Check sheet for the modelled part. Datum: model origin and axes. Units: mm. A direction names the side the tool comes from. Give positions to 0.01 mm unless a question says otherwise; leave off trailing zeros. Write each loop counter-clockwise with the first axis right and the second up, starting at its lowest first coordinate (ties: lowest second). Pieces come first, ordered by that corner, then holes. Notation, with made-up numbers: M 2,31 L 21,31 A38 ccw 21,70 Z; hole C 49,0.5 d4. An arc over 180 degrees is marked long. Use CSV: the item, a comma, the result in double quotes. Start each with the question number.
1. Cross-section at B-B, the plane z = -12.5. Enter the section's corners in (x, y).
2. Access from +Z, -Z, +X, -X, +Y, -Y to the whole of each face (thin tool, end or side, straight path). Record for faces 1 (the face through (0, 0, -1)), 2 (the face through (1, 2, 32.625)).
3. Cross-section at C-C, the plane y = 1.5. State how many separate pieces and enclosed holes the cut face has, and give its area (3 significant figures).
4. Scan lines: line 1 (X direction, y = 2, z = 35); line 2 (Z direction, x = 32, y = 2.05); line 3 (X direction, y = 1, z = 13.5). Record each from-to range of solid material in increasing order.
5. Mould release check, pull along Z, two halves, no side actions. Record for faces 3 (the face through (1, 1, -54.875)), 4 (the face through (51.36, 1.48, 50.85)), 5 (the face through (10.14, 1.52, -14.8)): +Z half, -Z half, draft (parallel to the pull), parting line (faces both ways), or undercut.
6. Cross-section at A-A, the plane z = -28.5. Enter the section's corners in (x, y), and give its area (3 significant figures).
from build123d import *

# Parameters (mm, degrees)
SKETCH1_R           = 3
BOSS_EXTRUDE1_DEPTH = 3
SKETCH2_W           = 28
SKETCH2_H           = 5
SKETCH2_W_2         = 35.5
CUT_EXTRUDE1_DEPTH  = 79.545892535
CUT_EXTRUDE2_DEPTH  = 79.545892535
FILLET1_R           = 1.5
SKETCH4_W           = 28
SKETCH4_H           = 5
CUT_EXTRUDE3_DEPTH  = 79.545892535


with BuildPart() as part:
    # Sketch1 → Boss-Extrude1 (new body)
    with BuildSketch(Plane(origin=(0, 0, 0), x_dir=(1, 0, 0), z_dir=(0, 1, 0))):
        with BuildLine():
            Line((55.872458647, -40.12463695), (55.872458647, 39.87536305))
            ThreePointArc((55.872458647, 39.87536305), (51.479060365, 50.481964768), (40.872458647, 54.87536305))
            Line((40.872458647, 54.87536305), (-39.127541353, 54.87536305))
            ThreePointArc((-39.127541353, 54.87536305), (-49.734143071, 50.481964768), (-54.127541353, 39.87536305))
            Line((-54.127541353, 39.87536305), (-54.127541353, -40.12463695))
            ThreePointArc((-54.127541353, -40.12463695), (-49.734143071, -50.731238667), (-39.127541353, -55.12463695))
            Line((-39.127541353, -55.12463695), (40.872458647, -55.12463695))
            ThreePointArc((40.872458647, -55.12463695), (51.479060365, -50.731238667), (55.872458647, -40.12463695))
        make_face()
        with Locations(Location((48.872458647, 32.87536305, 0), (0, 0, 270))):
            Circle(SKETCH1_R, mode=Mode.SUBTRACT)
        with Locations(Location((-47.127541353, -33.12463695, 0), (0, 0, 270))):
            Circle(SKETCH1_R, mode=Mode.SUBTRACT)
        with Locations(Location((-32.127541353, -48.12463695, 0), (0, 0, 270))):
            Circle(SKETCH1_R, mode=Mode.SUBTRACT)
        with Locations(Location((33.872458647, -48.12463695, 0), (0, 0, 270))):
            Circle(SKETCH1_R, mode=Mode.SUBTRACT)
        with Locations(Location((48.872458647, -33.12463695, 0), (0, 0, 270))):
            Circle(SKETCH1_R, mode=Mode.SUBTRACT)
        with Locations(Location((33.872458647, 47.87536305, 0), (0, 0, 270))):
            Circle(SKETCH1_R, mode=Mode.SUBTRACT)
        with Locations(Location((-32.127541353, 47.87536305, 0), (0, 0, 270))):
            Circle(SKETCH1_R, mode=Mode.SUBTRACT)
        with Locations(Location((-47.127541353, 32.87536305, 0), (0, 0, 270))):
            Circle(SKETCH1_R, mode=Mode.SUBTRACT)
    extrude(amount=BOSS_EXTRUDE1_DEPTH)

    # Sketch2 → Cut-Extrude1 (cut, through all)
    with BuildSketch(Plane(origin=(0, 3, 0), x_dir=(1, 0, 0), z_dir=(0, 1, 0))):
        with Locations((0.872458647, -35.12463695)):
            Rectangle(SKETCH2_W, SKETCH2_H)
        with Locations((0.872458647, 34.87536305)):
            Rectangle(SKETCH2_W_2, SKETCH2_H)
    extrude(amount=-CUT_EXTRUDE1_DEPTH, mode=Mode.SUBTRACT)

    # Sketch3 → Cut-Extrude2 (cut, through all)
    with BuildSketch(Plane(origin=(0, 3, 0), x_dir=(1, 0, 0), z_dir=(0, 1, 0))):
        Polygon((-39.127541353, 34.218508801), (-4.784395603, -0.12463695), (-39.127541353, -34.4677827), align=None)
        Polygon((-33.470687104, -40.12463695), (-21.127541353, -40.12463695), (-21.127541353, -27.781491199), align=None)
        Polygon((-33.470687104, 39.87536305), (-22.877541353, 39.87536305), (-22.877541353, 29.2822173), align=None)
        Polygon((40.872458647, -34.4677827), (40.872458647, 34.218508801), (6.529312896, -0.12463695), align=None)
        Polygon((24.622458647, 29.2822173), (24.622458647, 39.87536305), (35.215604397, 39.87536305), align=None)
        Polygon((-19.970687104, 26.37536305), (21.715604397, 26.37536305), (0.872458647, 5.5322173), align=None)
        Polygon((22.872458647, -40.12463695), (35.215604397, -40.12463695), (22.872458647, -27.781491199), align=None)
        Polygon((19.715604397, -24.62463695), (-17.970687104, -24.62463695), (0.872458647, -5.781491199), align=None)
    extrude(amount=-CUT_EXTRUDE2_DEPTH, mode=Mode.SUBTRACT)

    # Fillet1
    fillet1_edges = [part.edges().sort_by_distance(p)[0] for p in [
        (22.872458647, 1.5, 27.781491199),
        (-21.127541353, 1.5, 27.781491199),
        (24.622458647, 1.5, -29.2822173),
        (-19.970687104, 1.5, -26.37536305),
        (21.715604397, 1.5, -26.37536305),
        (19.715604397, 1.5, 24.62463695),
        (-17.970687104, 1.5, 24.62463695),
        (-22.877541353, 1.5, -29.2822173),
    ]]
    fillet(fillet1_edges, radius=FILLET1_R)

    # Sketch4 → Cut-Extrude3 (cut, through all)
    with BuildSketch(Plane(origin=(0, 3, 0), x_dir=(1, 0, 0), z_dir=(0, 1, 0))):
        with Locations((0.872458647, -48.12463695)):
            Rectangle(SKETCH4_W, SKETCH4_H)
    extrude(amount=-CUT_EXTRUDE3_DEPTH, mode=Mode.SUBTRACT)


solid = part.part
Worked answers:
1,outline,"M -54.13,0 L -39.13,0 L -39.13,3 L -54.13,3 Z; M -17.41,0 L -6.1,0 L -6.1,3 L -17.41,3 Z; M 7.84,0 L 19.15,0 L 19.15,3 L 7.84,3 Z; M 40.87,0 L 55.87,0 L 55.87,3 L 40.87,3 Z"
2,face 1,"+Z, -Z, +X, -X, -Y"
2,face 2,"+Y, -Y"
3,separate pieces,"1"
3,enclosed holes,"19"
3,area,"7,830 mm^2"
4,line 1,"x = -54.13 to -49.47, -44.79 to -28.35, -21.13 to -13.13, 14.87 to 22.87, 30.09 to 46.53, 51.21 to 55.87"
4,line 2,"z = -54.88 to -50.22, -45.53 to -39.88, -36.66 to -25.35, 25.6 to 36.91, 40.12 to 45.78, 50.47 to 55.12"
4,line 3,"x = -54.13 to -39.13, -18.16 to -6.85, 8.59 to 19.9, 40.87 to 55.87"
5,face 3,"-Z half"
5,face 4,"+Z half"
5,face 5,"undercut"
6,outline,"M -54.13,0 L -39.13,0 L -39.13,3 L -54.13,3 Z; M -33.41,0 L 35.15,0 L 35.15,3 L -33.41,3 Z; M 40.87,0 L 55.87,0 L 55.87,3 L 40.87,3 Z"
6,area,"296 mm^2"
